```python
from build123d import *

# Parameters (mm, degrees)
F1_DEPTH = 5
F3_DEPTH = 25
F4_W     = 42
F4_H     = 21
F4_W_2   = 13.2
F4_H_2   = 14.5
F5_DEPTH = 5.5


with BuildPart() as f1:
    # F0 (on Top) → F1 (new body)
    with BuildSketch(Plane.XY):
        Polygon((-90, 0), (-24.5, 0), (0, 22.5), (0, 135.5), (-114.5, 135.5), (-114.5, 22.5), align=None)
    extrude(amount=F1_DEPTH)

    # F2 (on face) → F3 (join)
    with BuildSketch(Plane.XY.offset(5)):
        Polygon((-114.5, 22.5), (-90, 0), (-24.5, 0), (0, 22.5), (0, 135.5), (-114.5, 135.5), align=None)
        Polygon((-5.5, 24.916429), (-26.642334, 5.5), (-87.857666, 5.5), (-109, 24.916429), (-109, 130), (-5.5, 130), align=None, mode=Mode.SUBTRACT)
    extrude(amount=F3_DEPTH)

    # F4 (on face) → F5 (cut, through all)
    with BuildSketch(Plane.YZ):
        with Locations((106.9, 15.5)):
            Rectangle(F4_W, F4_H)
        with Locations((63.3, 18.75)):
            Rectangle(F4_W_2, F4_H_2)
    extrude(amount=-F5_DEPTH, mode=Mode.SUBTRACT)


solid = f1.part
```
Check sheet for the modelled part. Datum: model origin and axes. Units: mm. A direction names the side the tool comes from. Round coordinates to 2 decimals unless told otherwise and drop trailing zeros. Write each loop counter-clockwise with the first axis right and the second up, starting at its lowest first coordinate (ties: lowest second). Pieces come first, ordered by that corner, then holes. Notation, with made-up numbers: (59, -15) -> (73, -15) arc R14 cw to (73, -10) -> close; hole circle Ø9 at (68.25, -26). An arc over 180 degrees is marked (long way). Put each result on its own line as item: value.
(1) Go/stop test with flat-tipped pins: pin 1 Ø4 at (x, y) = (-32.5, 56.5) entering from +Z; pin 2 Ø4.5 at (x, z) = (-4, 15.5) entering from -Y; pin 3 Ø3 at (x, z) = (-1.5, 19) entering from -Y. Record where each tip stops, or that it passes through.
Values found:
pin 1: stops at z = 5
pin 2: stops at y = 16.76
pin 3: stops at y = 19.74
(2) Sectioned sample at A-A (z = 27.75). Enter the section's corners in (x, y), plus the area to 3 significant figures.
Values found:
outline: (-114.5, 22.5) -> (-90, 0) -> (-24.5, 0) -> (0, 22.5) -> (0, 135.5) -> (-114.5, 135.5) -> close; hole (-109, 24.92) -> (-87.86, 5.5) -> (-26.64, 5.5) -> (-5.5, 24.92) -> (-5.5, 130) -> (-109, 130) -> close
area: 2,490 mm^2
(3) Sectioned sample at B-B (y = 123). Enter the section's corners in (x, z).
Values found:
outline: (-114.5, 0) -> (0, 0) -> (0, 5) -> (-109, 5) -> (-109, 30) -> (-114.5, 30) -> close; (-5.5, 26) -> (0, 26) -> (0, 30) -> (-5.5, 30) -> close
(4) Sectioned sample at D-D (y = 51). Enter the section's corners in (x, z), plus the area to 4 significant figures.
Values found:
outline: (-114.5, 0) -> (0, 0) -> (0, 30) -> (-5.5, 30) -> (-5.5, 5) -> (-109, 5) -> (-109, 30) -> (-114.5, 30) -> close
area: 847.5 mm^2
(5) Mould release check, pull along X, two halves, no side actions. Record for faces 4 (the face through (-57, 5.5, 17)), 5 (the face through (-102.422, 11.408, 14.79)), 6 (the face through (-3, 56.7, 19)): released by +X, released by -X, zero draft, split by the parting line, or undercut.
Values found:
face 4: undercut
face 5: released by -X
face 6: zero draft
(6) Sectioned sample at C-C (z = 19.75). Enter the section's corners in (x, y), plus the area to 3 significant figures.
Values found:
outline: (-114.5, 22.5) -> (-90, 0) -> (-24.5, 0) -> (0, 22.5) -> (0, 56.7) -> (-5.5, 56.7) -> (-5.5, 24.92) -> (-26.64, 5.5) -> (-87.86, 5.5) -> (-109, 24.92) -> (-109, 130) -> (-5.5, 130) -> (-5.5, 127.9) -> (0, 127.9) -> (0, 135.5) -> (-114.5, 135.5) -> close; (-5.5, 69.9) -> (0, 69.9) -> (0, 85.9) -> (-5.5, 85.9) -> close
area: 2,180 mm^2
(7) Material ranges on line 1 (Y direction, x = -74.5, z = 19); line 2 (X direction, y = 39, z = 22); line 3 (X direction, y = 121, z = 17.5), recorded low to high.
Values found:
line 1: y = 0 to 5.5, 130 to 135.5
line 2: x = -114.5 to -109, -5.5 to 0
line 3: x = -114.5 to -109
(8) Tool access check on faces 1 (the face through (-3, 69.9, 19)), 2 (the face through (-109, 77, 17)), 3 (the face through (-56, 135.5, 15)). Record the directions out of +Z, -Z, +X, -X, +Y, -Y that give a thin tool (end or side, any length) a straight path to the whole face; none if there is none.
Values found:
face 1: +X
face 2: +Z
face 3: +Z, -Z, +X, -X, +Y
